The listing builds one solid part. Answer for the finished solid, in the listing's coordinates (mm). Give positions to 0.01 mm unless a question says otherwise; leave off trailing zeros. Write each loop counter-clockwise with the first axis right and the second up, starting at its lowest first coordinate (ties: lowest second). Pieces come first, ordered by that corner, then holes. Notation, with made-up numbers: (-11.5, -14.5) - (13.5, -14.5) arc R16 cw to (13.5, 9.5) - close; hole circle Ø6 at (63.25, -23.75). An arc over 180 degrees is marked (long way). Answer as CSV lines item,"result". Start each with the question number.
(1) For a pull along X with two mould halves and no side action, classify faces 1 (the face through (0, 27, 2)), 2 (the face through (3.96, 52.73, 1.97)), 3 (the face through (6.396, 5.176, 1.972)), 4 (the face through (4, 28, 4)) as pulls with the +X half, pulls with the -X half, needs draft (parallel to the pull), parting line crosses it, or undercut.
(2) Find section A-A (y = 50.5). Write down the section's boundary in (x, z).
(3) Straight lines are drawn through the part: probe 1 along Y at (x, z) = (4.25, 1.65); probe 2 along Y at (x, z) = (2.25, 2.4); probe 3 along Y at (x, z) = (7.75, 3.5). For each, find the intervals that lie inside material, in ascending order.
(4) Find section C-C (z = 3.15). Write down the section's boundary in (x, y), then the cut area to 3 significant figures.
(5) Find section B-B (x = 2.5). Write down the section's boundary in (y, z).
from build123d import *

# Parameters (mm, degrees)
SKETCH_W  = 8.5
SKETCH_H  = 55
SKETCH_R  = 2.25
PAD_DEPTH = 4
FILLET_R  = 4


with BuildPart() as part:
    # Sketch → Pad (new body)
    with BuildSketch(Plane.XY):
        with Locations((4.25, 27.5)):
            Rectangle(SKETCH_W, SKETCH_H)
        with Locations((4.25, 4.5)):
            Circle(SKETCH_R, mode=Mode.SUBTRACT)
        with Locations((4.25, 50.5)):
            Circle(SKETCH_R, mode=Mode.SUBTRACT)
    extrude(amount=PAD_DEPTH)

    # Fillet
    fillet_edges = [part.edges().sort_by_distance(p)[0] for p in [
        (0, 55, 2),
        (8.5, 55, 2),
        (0, 0, 2),
        (8.5, 0, 2),
    ]]
    fillet(fillet_edges, radius=FILLET_R)


solid = part.part
Result set:
1,face 1,"pulls with the -X half"
1,face 2,"undercut"
1,face 3,"undercut"
1,face 4,"needs draft"
2,outline,"(0, 0) - (2, 0) - (2, 4) - (0, 4) - close; (6.5, 0) - (8.5, 0) - (8.5, 4) - (6.5, 4) - close"
3,probe 1,"0 to 2.25, 6.75 to 48.25, 52.75 to 55"
3,probe 2,"0.4 to 3.47, 5.53 to 49.47, 51.53 to 54.6"
3,probe 3,"1.67 to 53.33"
4,outline,"(0, 4) arc R4 ccw to (4, 0) - (4.5, 0) arc R4 ccw to (8.5, 4) - (8.5, 51) arc R4 ccw to (4.5, 55) - (4, 55) arc R4 ccw to (0, 51) - close; hole circle Ø4.5 at (4.25, 4.5); hole circle Ø4.5 at (4.25, 50.5)"
4,area,"422 mm^2"
5,outline,"(0.29, 0) - (3.09, 0) - (3.09, 4) - (0.29, 4) - close; (5.91, 0) - (49.09, 0) - (49.09, 4) - (5.91, 4) - close; (51.91, 0) - (54.71, 0) - (54.71, 4) - (51.91, 4) - close"
